Can you work these out from the model? Positions are in its coordinate system, mm. A direction names the side the tool comes from. Coordinates: 2 decimals unless noted, no trailing zeros. Loops run counter-clockwise (first coordinate to the right, second up) from the corner with the lowest first, then second, coordinate; pieces in that order, holes last. Notation, with made-up numbers: (15.5, 8.5) - (37.5, 8.5) arc R13 cw to (37.5, 25.5) - close; hole circle Ø9 at (74, 15.25). An arc over 180 degrees is marked (long way). Put each result on its own line as item: value. Start each with the question number.
from build123d import *

# Parameters (mm, degrees)
F0_R     = 45
F1_DEPTH = 60
F2_R     = 31
F3_DEPTH = 55
F4_R     = 25
F5_DEPTH = 25
F6_SIZE  = 1


with BuildPart() as f1:
    # F0 (on Front) → F1 (new body)
    with BuildSketch(Plane.XZ):
        Circle(F0_R)
    extrude(amount=F1_DEPTH)

    # F2 (on face) → F3 (cut)
    with BuildSketch(Plane.XZ.offset(60)):
        Circle(F2_R)
    extrude(amount=-F3_DEPTH, mode=Mode.SUBTRACT)

    # F4 (on face) → F5 (cut)
    with BuildSketch(Plane.XZ.offset(5)):
        Circle(F4_R)
    extrude(amount=-F5_DEPTH, mode=Mode.SUBTRACT)

    # F6
    f6_edges = [f1.edges().sort_by_distance(p)[0] for p in [
        (-45, -60, 0),
        (-31, -60, 0),
        (-45, 0, 0),
        (-25, 0, 0),
        (-25, -5, 0),
    ]]
    chamfer(f6_edges, length=F6_SIZE)


solid = f1.part
Q1. Please list where these lines run through material, in increasing order: line 1 along Z through (x, y) = (0, -41); line 2 along Z through (x, y) = (0, -2.8); line 3 along X through (y, z) = (-18, -6.5). Write a range as [from, to].
Q2. I want a section at A-A on x = 0. List the corners of the cut face in (y, z) for me.
Q3. On a 3-axis mill with a long thin cutter (end or side, diameter ignored), from which of +Z, -Z, +X, -X, +Y, -Y can I reach the whole of each face in a straight line? I mean faces 4 (the flat face through (-16, -5, -21)), 5 (the cylindrical face through (23.846, -2.521, 7.509)). Say none if no direction works.
Q4. Will these pins go through, and if not, where does the flat tip stop? pin 1 (6 mm diameter, centred on y = -51.5, z = -19.5, fed in from -X); pin 2 (1 mm diameter, centred on y = -16, z = 29.5, fed in from +X); pin 3 (18.5 mm diameter, centred on x = 5, z = -10.5, fed in from -Y); pin 4 (10 mm diameter, centred on x = 1, y = -22, fed in from +Z).
Q5. We'd pull the mould along X, two halves only. Please class faces 1 (the cylindrical face through (20.765, -29.594, -39.923)), 2 (the cylindrical face through (-4.036, -32.378, 30.736)), 3 (the flat face through (3.1, -60, -32.4)): released by +X, released by -X, zero draft, split by the parting line, or undercut.
Q6. I want a section at C-C on y = -6.5. List the corners of the cut face in (x, z) for me, and give its area (3 significant figures).
Q7. I want a section at B-B on z = 0. List the corners of the cut face in (x, y) for me.
Calculated:
1. line 1: [-45, -31], [31, 45]
1. line 2: [-45, -25], [25, 45]
1. line 3: [-44.53, -30.31], [30.31, 44.53]
2. outline: (-60, -44) - (-59, -45) - (-1, -45) - (0, -44) - (0, -26) - (-1, -25) - (-4, -25) - (-5, -26) - (-5, -31) - (-59, -31) - (-60, -32) - close; (-60, 32) - (-59, 31) - (-5, 31) - (-5, 26) - (-4, 25) - (-1, 25) - (0, 26) - (0, 44) - (-1, 45) - (-59, 45) - (-60, 44) - close
3. face 4: -Y
3. face 5: +Y, -Y
4. pin 1: x = -41.87
4. pin 2: x = 34.41
4. pin 3: through
4. pin 4: z = 45
5. face 1: split by the parting line
5. face 2: undercut
5. face 3: zero draft
6. outline: circle Ø90 at (0, 0); hole circle Ø62 at (0, 0)
6. area: 3,340 mm2
7. outline: (-45, -59) - (-44, -60) - (-32, -60) - (-31, -59) - (-31, -5) - (-26, -5) - (-25, -4) - (-25, -1) - (-26, 0) - (-44, 0) - (-45, -1) - close; (25, -4) - (26, -5) - (31, -5) - (31, -59) - (32, -60) - (44, -60) - (45, -59) - (45, -1) - (44, 0) - (26, 0) - (25, -1) - close
